The listing builds one solid part. Answer for the finished solid, in the listing's coordinates (mm). A direction names the side the tool comes from. Round coordinates to 2 decimals unless told otherwise and drop trailing zeros. Write each loop counter-clockwise with the first axis right and the second up, starting at its lowest first coordinate (ties: lowest second). Pieces come first, ordered by that corner, then holes.
from build123d import *

# Parameters (mm, degrees)
SKETCH_R           = 1.8
PAD_DEPTH          = 5.2
SKETCH002_R        = 11
SKETCH002_R_2      = 1.5
PAD001_DEPTH       = 8
SKETCH003_R        = 7.3
POCKET001_DEPTH    = 5.2
POCKET_DEPTH       = 10.5
SKETCH005_R        = 1.75
POCKET002_DEPTH    = 28.451
SKETCH006_W        = 6
SKETCH006_H        = 3
POCKET003_DEPTH    = 8
SKETCH007_R        = 1.2
PAD002_DEPTH       = 5.2
SKETCH008_W        = 4.5
SKETCH008_H        = 15
POCKET004_DEPTH    = 1
POLARPATTERN_COUNT = 3


with BuildPart() as part:
    # Sketch → Pad (new body)
    with BuildSketch(Plane.XY):
        with BuildLine():
            Line((-14.982239, -3.65), (-4.330127, 14.8))
            ThreePointArc((4.330127, 14.8), (0, 17.3), (-4.330127, 14.8))
            Line((4.330127, 14.8), (14.982239, -3.65))
            ThreePointArc((10.652112, -11.15), (14.982239, -8.65), (14.982239, -3.65))
            Line((10.652112, -11.15), (-10.652112, -11.15))
            ThreePointArc((-14.982239, -3.65), (-14.982239, -8.65), (-10.652112, -11.15))
        make_face()
        with Locations((0, 12.3)):
            Circle(SKETCH_R, mode=Mode.SUBTRACT)
        with Locations((-10.652112, -6.15)):
            Circle(SKETCH_R, mode=Mode.SUBTRACT)
        with Locations((10.652112, -6.15)):
            Circle(SKETCH_R, mode=Mode.SUBTRACT)
    extrude(amount=PAD_DEPTH)

    # Sketch002 (on Face11 of Pad) → Pad001 (join)
    with BuildSketch(Plane.XY.offset(5.2)):
        Circle(SKETCH002_R)
        Circle(SKETCH002_R_2, mode=Mode.SUBTRACT)
    extrude(amount=PAD001_DEPTH)

    # Sketch003 (on Face4 of Pad001) → Pocket001 (cut)
    with BuildSketch(Plane(origin=(0, 0, 0), x_dir=(1, 0, 0), z_dir=(0, 0, -1))):
        Circle(SKETCH003_R)
    extrude(amount=-POCKET001_DEPTH, mode=Mode.SUBTRACT)

    # Sketch004 (on Face18 of Pocket001) → Pocket (cut)
    with BuildSketch(Plane.XY.offset(13.2)):
        Polygon((-7.188011, -6.15), (-8.920062, -3.15), (-12.384163, -3.15), (-14.116214, -6.15), (-12.384163, -9.15), (-8.920062, -9.15), align=None)
        Polygon((1.732051, 9.3), (3.464102, 12.3), (1.732051, 15.3), (-1.732051, 15.3), (-3.464102, 12.3), (-1.732051, 9.3), align=None)
        Polygon((12.384163, -9.15), (14.116214, -6.15), (12.384163, -3.15), (8.920062, -3.15), (7.188011, -6.15), (8.920062, -9.15), align=None)
    extrude(amount=-POCKET_DEPTH, mode=Mode.SUBTRACT)

    # Sketch005 (on Face6 of Pocket) → Pocket002 (cut, through all)
    with BuildSketch(Plane.XZ.offset(11.15)):
        with Locations((0, 9)):
            Circle(SKETCH005_R)
    extrude(amount=-POCKET002_DEPTH, mode=Mode.SUBTRACT)

    # Sketch006 (on Face36 of Pocket002) → Pocket003 (cut)
    with BuildSketch(Plane.XY.offset(13.2)):
        with Locations((0, 5)):
            Rectangle(SKETCH006_W, SKETCH006_H)
        with Locations((0, -5)):
            Rectangle(SKETCH006_W, SKETCH006_H)
    extrude(amount=-POCKET003_DEPTH, mode=Mode.SUBTRACT)

    # Sketch007 (on Face33 of Pocket003) → Pad002 (join)
    with BuildSketch(Plane(origin=(0, 0, 5.2), x_dir=(1, 0, 0), z_dir=(0, 0, -1))):
        with BuildLine():
            Line((-1.346291, 3.5), (1.346291, 3.5))
            ThreePointArc((1.346291, -3.5), (3.75, 0), (1.346291, 3.5))
            Line((1.346291, -3.5), (-1.346291, -3.5))
            ThreePointArc((-1.346291, 3.5), (-3.75, 0), (-1.346291, -3.5))
        make_face()
        Circle(SKETCH007_R, mode=Mode.SUBTRACT)
    extrude(amount=PAD002_DEPTH)

    # Sketch008 (on Face4 of Pad002) → Pocket004 (cut)
    with BuildSketch(Plane(origin=(0, 0, 0), x_dir=(1, 0, 0), z_dir=(0, 0, -1))):
        with Locations((0, -11.3)):
            Rectangle(SKETCH008_W, SKETCH008_H)
    pocket004 = extrude(amount=-POCKET004_DEPTH, mode=Mode.SUBTRACT)

    # PolarPattern: Pocket004 ×3 about axis
    polarpattern_axis = Axis((0, 0, 0), (0, 0, -1))
    for i in range(1, POLARPATTERN_COUNT):
        add(pocket004.rotate(polarpattern_axis, i * 360 / POLARPATTERN_COUNT), mode=Mode.SUBTRACT)


solid = part.part
1. Section D-D on x = 0 is taken. Give the number of separate pieces and of enclosed holes in the cut face, plus the area to 3 significant figures.
Geometry says:
separate pieces: 9
enclosed holes: 0
area: 116 mm2
2. Straight lines are drawn through the part: line 1 along Y through (x, z) = (0, 1.85); line 2 along X through (y, z) = (-5.25, 3.25); line 3 along X through (y, z) = (-6.15, 2.3). For each, find the intervals that lie inside material, in ascending order.
Geometry says:
line 1: y = -11.15 to -7.3, -3.5 to -1.2, 1.2 to 3.5, 7.3 to 10.5, 14.1 to 17.3
line 2: x = -15.57 to -13.6, -7.71 to -5.07, 5.07 to 7.71, 13.6 to 15.57
line 3: x = -15.65 to -12.45, -8.85 to -3.93, 3.93 to 8.85, 12.45 to 15.65
3. Given pin 1 (0.9 mm diameter, centred on y = -5, z = 8, fed in from +X); pin 2 (5 mm diameter, centred on y = 5, z = 2, fed in from -X); pin 3 (0.8 mm diameter, centred on y = 10, z = 0.5, fed in from -X), each flat-ended and moving along its own axis, determine where each tip first touches the part or whether it passes through.
Geometry says:
pin 1: stops at x = 8.11
pin 2: stops at x = -11.43
pin 3: stops at x = -7.33
4. Section C-C on z = 11.25 is taken. Determine the outline of the cut face in (x, y).
Geometry says:
outline: (-10.54, -3.15) - (-8.92, -3.15) - (-7.19, -6.15) - (-8, -7.55) arc R11 ccw to (8, -7.55) - (7.19, -6.15) - (8.92, -3.15) - (10.54, -3.15) arc R11 ccw to (2.54, 10.7) - (1.73, 9.3) - (-1.73, 9.3) - (-2.54, 10.7) arc R11 ccw to start; hole (-3, -6.5) - (3, -6.5) - (3, -3.5) - (-3, -3.5) - close; hole (-3, 3.5) - (3, 3.5) - (3, 6.5) - (-3, 6.5) - close; hole circle Ø3 at (0, 0)
5. For a pull along Y with two mould halves and no side action, classify faces 1 (the face through (10, -3.15, 7)), 2 (the face through (-8.7, -6.8, 1)), 3 (the face through (2.25, 11.9, 0.5)), 4 (the face through (-15.018, -8.586, 2.564)) as released by +Y, released by -Y, zero draft, split by the parting line, or undercut.
Geometry says:
face 1: undercut
face 2: undercut
face 3: zero draft
face 4: split by the parting line
6. Section B-B on y = 0 is taken. Determine the outline of the cut face in (x, z).
Geometry says:
outline: (-12.87, 0) - (-7.3, 0) - (-7.3, 5.2) - (-3.75, 5.2) - (-3.75, 0) - (-1.2, 0) - (-1.2, 5.2) - (-1.5, 5.2) - (-1.5, 8.1) arc R1.75 cw to (-1.5, 9.9) - (-1.5, 13.2) - (-11, 13.2) - (-11, 5.2) - (-12.87, 5.2) - close; (1.2, 0) - (3.75, 0) - (3.75, 5.2) - (7.3, 5.2) - (7.3, 0) - (12.87, 0) - (12.87, 5.2) - (11, 5.2) - (11, 13.2) - (1.5, 13.2) - (1.5, 9.9) arc R1.75 cw to (1.5, 8.1) - (1.5, 5.2) - (1.2, 5.2) - close
7. A tool of negligible diameter and unlimited length cuts with its end or side. For faces 5 (the face through (0, -11, 11)), 6 (the face through (-2, 11, 1)), 7 (the face through (6.963, -2.193, 2.564)), 8 (the face through (-11, -9.15, 4)), from which of +Z, -Z, +X, -X, +Y, -Y can it reach the whole face along a straight path? Write none if from no direction.
Geometry says:
face 5: +Z, -Y
face 6: -Z, +Y
face 7: -Z
face 8: +Z
8. Section A-A on z = 1.75 is taken. Determine the outline of the cut face in (x, y).
Geometry says:
outline: (-14.98, -3.65) arc R5 ccw to (-10.65, -11.15) - (10.65, -11.15) arc R5 ccw to (14.98, -3.65) - (4.33, 14.8) arc R5 ccw to (-4.33, 14.8) - close; (-1.35, -3.5) - (1.35, -3.5) arc R3.75 ccw to (1.35, 3.5) - (-1.35, 3.5) arc R3.75 ccw to start; hole circle Ø3.6 at (-10.65, -6.15); hole circle Ø14.6 at (0, 0); hole circle Ø3.6 at (0, 12.3); hole circle Ø2.4 at (0, 0); hole circle Ø3.6 at (10.65, -6.15)
